CAD build for the part. Positions are in the model's coordinates, mm. Give positions to 0.01 mm unless a question says otherwise; leave off trailing zeros. Write each loop counter-clockwise with the first axis right and the second up, starting at its lowest first coordinate (ties: lowest second). Pieces come first, ordered by that corner, then holes. Notation, with made-up numbers: (14, 61) - (50, 61) arc R8 cw to (50, 73) - close; hole circle Ø8 at (10.5, -21.75). An arc over 180 degrees is marked (long way). Put each result on its own line as item: value. Start each with the question number.
1. Drop a flat-ended pin along its axis: pin 1 (1 mm diameter, centred on x = 11.5, y = 1, fed in from -Z). Give the stop position or say it passes through.
2. Cut at A-A on x = -4. List the corners of the cut face in (y, z).
3. Wall check: line 1 (Z direction, x = -12, y = -1.3); line 2 (Z direction, x = 13.75, y = 0.15); line 3 (X direction, y = 1.7, z = -0.5). Give the ranges that are in metal, low to high.
Autodesk Inventor part; units mm, degrees
ref_plane "YZ Plane" through (0, 0, 0) normal (1, 0, 0) x (0, 1, 0)
ref_plane "XZ Plane" through (0, 0, 0) normal (0, 1, 0) x (-1, 0, 0)
ref_plane "XY Plane" through (0, 0, 0) normal (0, 0, 1) x (1, 0, 0)
sketch "Sketch1" plane through (0, 0, 0) normal (1, 0, 0) x (0, 1, 0)
  line L0 (0, 9.9) -> (0, -9.9) construction
  line L1 (-1.95, 9.9) -> (-1.95, -9.9)
  line L2 (1.95, -9.9) -> (1.95, 9.9)
  arc A0 (1.95, 9.9) -> (-1.95, 9.9) centre (0, 9.9) ccw
  arc A1 (-1.95, -9.9) -> (1.95, -9.9) centre (0, -9.9) ccw
  point P0 (0, 0)
  dimension "d0" = 9.9
  dimension "d1" = 3.9
extrude "Extrusion1" add sketch "Sketch1" along normal mid plane 30
chamfer "Chamfer1" distance 0.5 angle 45 8 edges at (-15, 1.95, 0) (-15, 0, -11.85) (-15, -1.95, 0) (-15, 0, 11.85) (15, 1.95, 0) (15, 0, 11.85) (15, -1.95, 0) (15, 0, -11.85)
properties part number "Domino2"
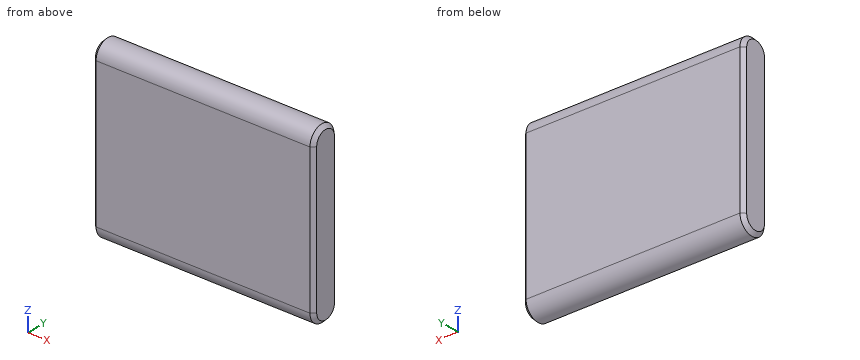
Report:
1. pin 1: stops at z = -11.78
2. outline: (-1.95, -9.9) arc R1.95 ccw to (1.95, -9.9) - (1.95, 9.9) arc R1.95 ccw to (-1.95, 9.9) - close
3. line 1: z = -11.35 to 11.35
3. line 2: z = -11.84 to 11.84
3. line 3: x = -14.75 to 14.75
